Could you check a few things on this drawing? It's one solid part, dimensions in mm from its lowest x, y, z. Round coordinates to 2 decimals unless told otherwise and drop trailing zeros. Loops run counter-clockwise (first coordinate to the right, second up) from the corner with the lowest first, then second, coordinate; pieces in that order, holes last. Notation, with made-up numbers: M 44,-2 L 65,-2 A9 cw 65,4 Z; hole C -17.5,85.5 d5. An arc over 180 degrees is marked long. Return JSON: item names as keys, results as strings.
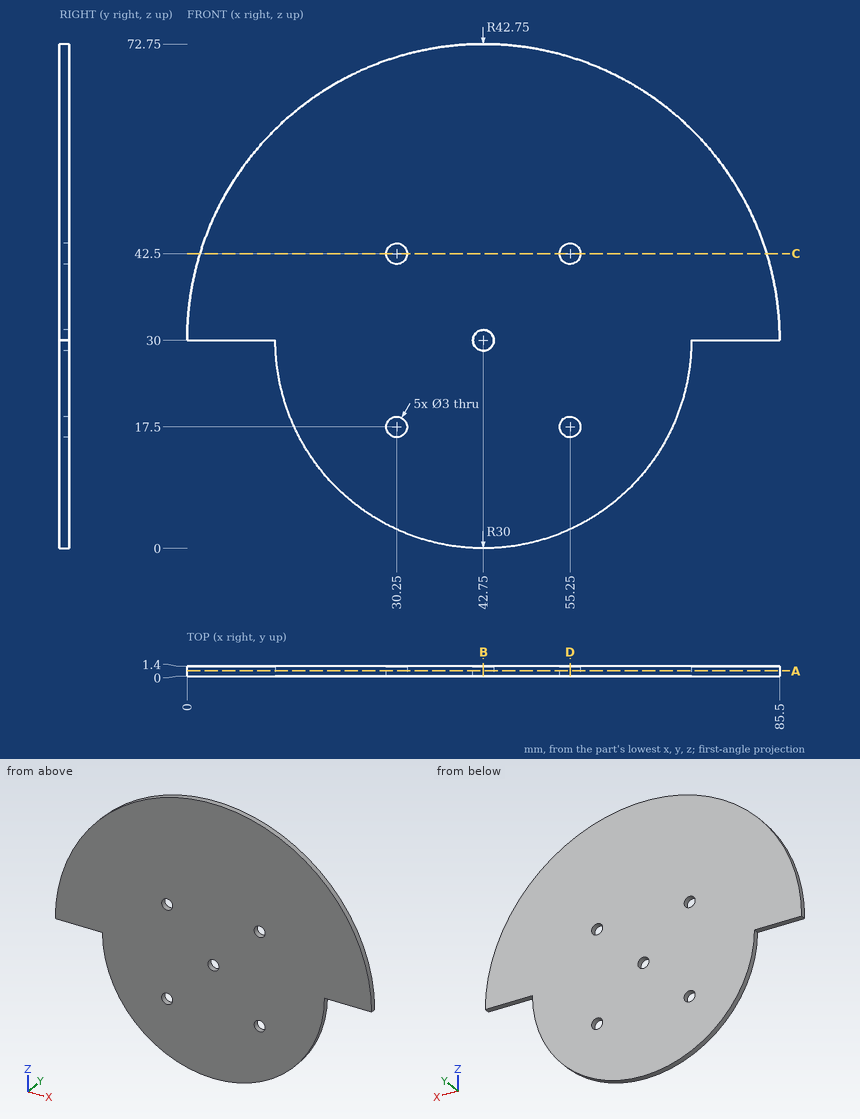
Q1. Suppose I cut it at D-D, the plane x = 55.25. Please give me the cut outline in (y, z), plus the area to 3 significant figures.
Results:
{"outline": "M 0,2.73 L 1.4,2.73 L 1.4,16 L 0,16 Z; M 0,19 L 1.4,19 L 1.4,41 L 0,41 Z; M 0,44 L 1.4,44 L 1.4,70.88 L 0,70.88 Z", "area": "87.0 mm2"}
Q2. Suppose I cut it at A-A, the plane y = 0.75. Please give me the cut outline in (x, z), plus the area to 3 significant figures.
Results:
{"outline": "M 0,30 L 12.75,30 A30 ccw 72.75,30 L 85.5,30 A42.75 ccw Z; hole C 30.25,17.5 d3; hole C 30.25,42.5 d3; hole C 42.75,30 d3; hole C 55.25,17.5 d3; hole C 55.25,42.5 d3", "area": "4,250 mm2"}
Q3. I'm going to push a flat-ended pin straight in: pin 1 Ø2.5 at (x, z) = (55.25, 17.5) entering from -Y. Where does the tip first touch, or does it pass through?
Results:
{"pin 1": "passes through"}
Q4. Suppose I cut it at B-B, the plane x = 42.75. Please give me the cut outline in (y, z).
Results:
{"outline": "M 0,0 L 1.4,0 L 1.4,28.5 L 0,28.5 Z; M 0,31.5 L 1.4,31.5 L 1.4,72.75 L 0,72.75 Z"}
Q5. If I drill on line 1 along Z through (x, y) = (30.25, 0.55); line 2 along Z through (x, y) = (42.75, 0.85); line 3 along X through (y, z) = (1, 29.5), over which ranges is the centre line in solid material (lowest first)?
Results:
{"line 1": "z = 2.73 to 16, 19 to 41, 44 to 70.88", "line 2": "z = 0 to 28.5, 31.5 to 72.75", "line 3": "x = 12.75 to 41.34, 44.16 to 72.75"}
Q6. Suppose I cut it at C-C, the plane z = 42.5. Please give me the cut outline in (x, y).
Results:
{"outline": "M 1.87,0 L 28.75,0 L 28.75,1.4 L 1.87,1.4 Z; M 31.75,0 L 53.75,0 L 53.75,1.4 L 31.75,1.4 Z; M 56.75,0 L 83.63,0 L 83.63,1.4 L 56.75,1.4 Z"}
